Input: part model. Units: mm. Frame: model coordinates. A direction names the side the tool comes from. Give positions to 0.01 mm unless a question says otherwise; leave off trailing zeros. Loops run counter-clockwise (first coordinate to the right, second up) from the corner with the lowest first, then second, coordinate; pieces in that order, holes last. Notation, with made-up numbers: M 78.5,50 L 94.5,50 A21 cw 94.5,79 Z; hole C 74.25,-34 d8. An arc over 180 degrees is marked long. Use a Markdown table: item, result. Add a question column.
Autodesk Inventor part; units mm, degrees
ref_plane "YZ Plane" through (0, 0, 0) normal (1, 0, 0) x (0, 1, 0)
ref_plane "XZ Plane" through (0, 0, 0) normal (0, 1, 0) x (-1, 0, 0)
ref_plane "XY Plane" through (0, 0, 0) normal (0, 0, 1) x (1, 0, 0)
sketch "Esboço1" plane through (0, 0, 0) normal (0, 1, 0) x (-1, 0, 0)
  line L0 (-59, 59) -> (59, 59)
  line L1 (59, 59) -> (59, -59)
  line L2 (59, -59) -> (-59, -59)
  line L3 (-59, -59) -> (-59, 59)
  line L4 (-59, 59) -> (59, -59) construction
  line L5 (59, 59) -> (-59, -59) construction
  point P0 (0, 0)
  dimension "d0" = 118
  dimension "d1" = 118
extrude "Extrusão1" add sketch "Esboço1" along normal blind 4
sketch "Esboço2" plane through (0, 0, 0) normal (0, -1, 0) x (1, 0, 0)
  line L0 (-52, -52) -> (40, -52)
  line L1 (52, -40) -> (52, 52)
  line L2 (52, 52) -> (-40, 52)
  line L3 (-52, 40) -> (-52, -52)
  line L4 (-52, -52) -> (52, 52) construction
  line L5 (52, -52) -> (-52, 52) construction
  line L6 (-40, 52) -> (-40, 44)
  line L7 (-44, 40) -> (-52, 40)
  line L8 (40, -52) -> (40, -44)
  line L9 (44, -40) -> (52, -40)
  arc A0 (-44, 40) -> (-40, 44) centre (-44, 44) ccw
  arc A1 (44, -40) -> (40, -44) centre (44, -44) ccw
  point P0 (0, 0)
  dimension "d13" = 4
extrude "Extrusão2" add sketch "Esboço2" along normal blind 4
fillet "Arredondamento1" radius 2 4 edges at (59, 2, 59) (59, 2, -59) (-59, 2, 59) (-59, 2, -59)
sketch "Esboço3" plane through (0, 0, 0) normal (0, -1, 0) x (1, 0, 0)
  circle A0 centre (53, -53) radius 2.005
  circle A1 centre (-53, 53) radius 2.005
  line L0 (57, -59) -> (-57, -59)
  line L1 (59, 57) -> (59, -57)
  line L2 (-59, -57) -> (-59, 57)
  line L3 (-57, 59) -> (57, 59)
  point P0 (0, 0)
  dimension "d15" = 4.01
  dimension "d16" = 4.01
  dimension "d17" = 6
  dimension "d18" = 6
  dimension "d19" = 6
  dimension "d20" = 6
extrude "Extrusão3" cut sketch "Esboço3" against normal blind 4
properties part number "tampa caixa"
1) Pull-direction query (X, two-part tool) for faces 6 (the cylindrical face through (-55.003, 1.972, 53.088)), 7 (the flat face through (7, -2, 52)), 8 (the cylindrical face through (-41.141, -1.972, 41.203)); classes: pulls with the +X half, pulls with the -X half, needs draft (parallel to the pull), parting line crosses it, or undercut.
2) Ray query, line 1 (Z direction, x = -13, y = -3.5); line 2 (X direction, y = -3.25, z = -44.5). Return the intervals inside material, ascending. Write a range as [from, to].
3) Contact query for flat-ended pins moving along their axis: P1, Ø1.2, axis at y = -2.5, z = -28.5, coming from the -X side; P2, Ø1.2, axis at y = -2, z = 50, coming from the -X side; P3, Ø1.2, axis at y = -2.5, z = 26, coming from the +X side. Output: stop coordinate, or through.
4) Section query A-A, the plane z = -16. Return the cut outline in (x, y), and give its area (3 significant figures).
5) Reachability of faces 1 (the flat face through (-52, -2, -5)), 2 (the flat face through (52, -2, 5)), 3 (the flat face through (-7, -2, -52)), 4 (the flat face through (40, -2, -48)), 5 (the flat face through (-48, -2, 40)) from +Z, -Z, +X, -X, +Y, -Y: full face, straight path, thin tool, end or side. Return the list, or none.
6) Section query C-C, the plane x = 35. Return the cut outline in (y, z), and give its area (3 significant figures).
7) Section query B-B, the plane y = -2.5. Return the cut outline in (x, z), and give its area (3 significant figures).
Entries:
| question | item | result |
|---|---|---|
| 1 | face 6 | undercut |
| 1 | face 7 | needs draft |
| 1 | face 8 | pulls with the -X half |
| 2 | line 1 | z = [-52, 52] |
| 2 | line 2 | x = [-52, 40] |
| 3 | P1 | stops at x = -52 |
| 3 | P2 | stops at x = -40 |
| 3 | P3 | stops at x = 52 |
| 4 | outline | M -59,0 L -52,0 L -52,-4 L 52,-4 L 52,0 L 59,0 L 59,4 L -59,4 Z |
| 4 | area | 888 mm² |
| 5 | face 1 | +Z, -Z, -X, -Y |
| 5 | face 2 | +Z, -Z, +X, -Y |
| 5 | face 3 | -Z, +X, -X, -Y |
| 5 | face 4 | -Z, +X, -Y |
| 5 | face 5 | +Z, -X, -Y |
| 6 | outline | M -4,-52 L 0,-52 L 0,-59 L 4,-59 L 4,59 L 0,59 L 0,52 L -4,52 Z |
| 6 | area | 888 mm² |
| 7 | outline | M -52,-52 L 40,-52 L 40,-44 A4 cw 44,-40 L 52,-40 L 52,52 L -40,52 L -40,44 A4 cw -44,40 L -52,40 Z |
| 7 | area | 10,500 mm² |
